from build123d import *

# Parameters (mm, degrees)
F0_W     = 302.65603
F0_H     = 461.279019
F1_DEPTH = 19.05
F2_W     = 45.347571
F2_H     = 50.879955
F2_W_2   = 45.347572
F2_H_2   = 50.879956
F3_DEPTH = 762


with BuildPart() as f1:
    # F0 (on Top) → F1 (new body)
    with BuildSketch(Plane.XY):
        with Locations((102.108258, 177.309223)):
            Rectangle(F0_W, F0_H)
    extrude(amount=F1_DEPTH)

    # F2 (on Top) → F3 (join)
    with BuildSketch(Plane.XY):
        with Locations((229.558259, -25.439977)):
            Rectangle(F2_W, F2_H)
        Rectangle(F2_W_2, F2_H_2)
    extrude(amount=-F3_DEPTH)


solid = f1.part
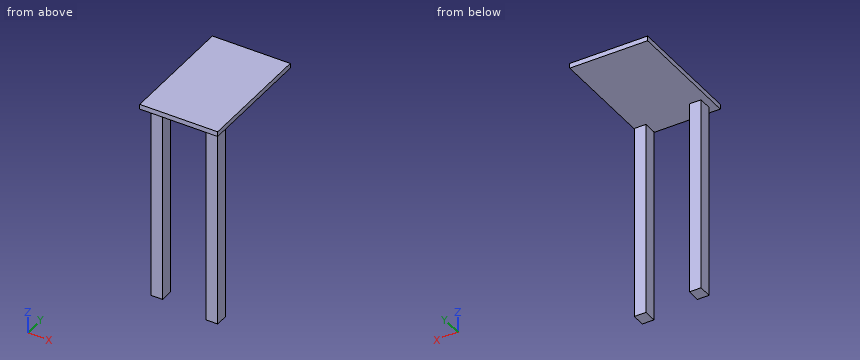
Build history of the part. All positions in model axes, mm. Coordinates: 2 decimals unless noted, no trailing zeros. Write each loop counter-clockwise with the first axis right and the second up, starting at its lowest first coordinate (ties: lowest second). Pieces come first, ordered by that corner, then holes.
(1) Cut at D-D on x = 102.5. List the corners of the cut face in (y, z), and give its area (3 significant figures).
(2) Cut at A-A on z = -355. List the corners of the cut face in (x, y), and give its area (3 significant figures).
(3) Drill centre lines: line 1 (X direction, y = -24, z = -449); line 2 (Y direction, x = 236, z = -70.5); line 3 (Z direction, x = 141.5, y = 279). Where is each one in solid material? Low to high.
(4) Cut at B-B on y = -8.5. List the corners of the cut face in (x, z), and give its area (3 significant figures).
(5) Cut at C-C on x = 215. List the corners of the cut face in (y, z).
(6) Pin check, flat tips, straight feed: pin 1 Ø4 at (x, y) = (-14.5, 268.5) entering from -Z; pin 2 Ø22.5 at (x, z) = (220.5, -361.5) entering from -Y; pin 3 Ø13.5 at (x, z) = (7.5, -311.5) entering from -Y. Stop position of each tip, or through.
Working result:
1. outline: (-53.33, 0) - (407.95, 0) - (407.95, 19.05) - (-53.33, 19.05) - close
1. area: 8,790 mm2
2. outline: (-22.67, -25.44) - (22.67, -25.44) - (22.67, 25.44) - (-22.67, 25.44) - close; (206.88, -50.88) - (252.23, -50.88) - (252.23, 0) - (206.88, 0) - close
2. area: 4,610 mm2
3. line 1: x = -22.67 to 22.67, 206.88 to 252.23
3. line 2: y = -50.88 to 0
3. line 3: z = 0 to 19.05
4. outline: (-49.22, 0) - (-22.67, 0) - (-22.67, -762) - (22.67, -762) - (22.67, 0) - (206.88, 0) - (206.88, -762) - (252.23, -762) - (252.23, 0) - (253.44, 0) - (253.44, 19.05) - (-49.22, 19.05) - close
4. area: 74,900 mm2
5. outline: (-53.33, 0) - (-50.88, 0) - (-50.88, -762) - (0, -762) - (0, 0) - (407.95, 0) - (407.95, 19.05) - (-53.33, 19.05) - close
6. pin 1: stops at z = 0
6. pin 2: stops at y = -50.88
6. pin 3: stops at y = -25.44
